The model under review builds one solid part; all positions refer to its coordinate system, in mm. A direction names the side the tool comes from. Coordinates: 2 decimals unless noted, no trailing zeros. Write each loop counter-clockwise with the first axis right and the second up, starting at its lowest first coordinate (ties: lowest second). Pieces come first, ordered by that corner, then holes. Notation, with made-up numbers: (84.5, 67.5) - (125.5, 67.5) arc R17 cw to (125.5, 86.5) - close; hole circle Ø7 at (-28.75, 41.5). An arc over 180 degrees is marked (long way). Put each result on its own line as item: value. Start each with the question number.
Item 1: Machinability: for faces 5 (the face through (-0.867, 3.905, -29.371)), 6 (the face through (-0.058, 0.466, -38.022)), 7 (the face through (0, 0, 10.5)), 8 (the face through (-0.867, -3.905, 6.444)), 9 (the face through (6.026, 10.438, 6.444)), which of the approach directions +Z, -Z, +X, -X, +Y, -Y give a long, thin tool a straight path to every point of the face, cutting with its end or side? Answer none if there is none.
Item 2: To check wall thickness, follow L1, parallel to Z at x = 0.5, y = 0; L2, parallel to Y at x = -0.25, z = -39.5; L3, parallel to Z at x = 4, y = 11.5. State the ranges of each line that lie inside material, in increasing order. Write a range as [from, to].
Item 3: Consider section A-A on y = 0. Give the boundary of the cut face in (x, z), then the cut area to 3 significant figures.
Item 4: Consider section D-D on z = -39.5. Give the boundary of the cut face in (x, y), then the cut area to 3 significant figures.
Item 5: Consider section C-C on z = -9.5. Give the boundary of the cut face in (x, y).
Item 6: Mouldability with a two-part tool opening along X and no side actions: class faces 1 (the face through (-5.974, 10.347, 6.444)), 2 (the face through (0.06, 8.25, 6.44)), 3 (the face through (-0.12, 15.75, 6.44)), 4 (the face through (0, 0, -55.5)) as pulls with the +X half, pulls with the -X half, needs draft (parallel to the pull), parting line crosses it, or undercut.
Item 7: Consider section B-B on x = 0. Give the boundary of the cut face in (y, z), then the cut area to 3 significant figures.
Item 8: For pin 1 (4 mm diameter, centred on x = 8, y = -0.5, fed in from +Z); pin 2 (6 mm diameter, centred on y = -4.5, z = 4, fed in from +X); pin 3 (8 mm diameter, centred on x = 6.5, z = -13, fed in from +Y), all flat-tipped, find the tip position at first contact; note any pin that passes through.
```python
from build123d import *

# Parameters (mm, degrees)
SKETCH1_R                           = 17.5
BOSS_EXTRUDE1_DEPTH                 = 2.5
BOSS_EXTRUDE2_DEPTH                 = 8
SKETCH3_R                           = 4
BOSS_EXTRUDE3_DEPTH                 = 8
BOSS_EXTRUDE4_START                 = 53
SKETCH7_R                           = 4
BOSS_EXTRUDE4_DEPTH                 = 53
CUT_EXTRUDE1_REACH                  = 62.768
CUT_EXTRUDE1_END_RADIUS             = 4
SKETCH8_R                           = 1.55
CUT_EXTRUDE1_DIRECTION_2_REACH      = 62.768
CUT_EXTRUDE1_DIRECTION_2_END_RADIUS = 4


with BuildPart() as part:
    # Sketch1 → Boss-Extrude1 (new, symmetric)
    with BuildSketch(Plane.XY):
        Circle(SKETCH1_R)
    extrude(amount=BOSS_EXTRUDE1_DEPTH, both=True)

    # Sketch2 → Boss-Extrude2 (add)
    with BuildSketch(Plane.XY.offset(2.5)):
        with BuildLine():
            Line((7.875, 13.63990011), (4.125, 7.144709581))
            ThreePointArc((4.125, 7.144709581), (0, 8.25), (-4.125, 7.144709581))
            Line((-4.125, 7.144709581), (-7.875, 13.63990011))
            ThreePointArc((-7.875, 13.63990011), (0, 15.75), (7.875, 13.63990011))
        make_face()
    extrude(amount=BOSS_EXTRUDE2_DEPTH)

    # Sketch3 → Boss-Extrude3 (add)
    with BuildSketch(Plane.XY.offset(2.5)):
        Circle(SKETCH3_R)
    extrude(amount=BOSS_EXTRUDE3_DEPTH)

    # Sketch7 → Boss-Extrude4 (add)
    with BuildSketch(Plane(origin=(0, 0, -2.5), x_dir=(-1, 0, 0), z_dir=(0, 0, -1)).offset(BOSS_EXTRUDE4_START)):
        with Locations(Location((0, 0, 0), (0, 0, 180))):
            Circle(SKETCH7_R)
    extrude(amount=-BOSS_EXTRUDE4_DEPTH)

    # Cut-Extrude1: up to this cylinder (the profile starts inside it)
    cut_extrude1_end = Plane(origin=(0, 0, -39.5), z_dir=(0, 0, 1)) * Cylinder(CUT_EXTRUDE1_END_RADIUS, 134.536, mode=Mode.PRIVATE)
    # Sketch8 → Cut-Extrude1 (cut, up to the surface)
    with BuildSketch(Plane.ZY, mode=Mode.PRIVATE) as cut_extrude1_sk1:
        with Locations((-39.5, 0)):
            Circle(SKETCH8_R)
    cut_extrude1_tool1 = extrude(cut_extrude1_sk1.sketch, amount=-CUT_EXTRUDE1_REACH, mode=Mode.PRIVATE) & cut_extrude1_end
    add(cut_extrude1_tool1.solids().sort_by_distance((0, 0, -39.5))[0], mode=Mode.SUBTRACT)

    # Cut-Extrude1 direction 2: up to this cylinder (the profile starts inside it)
    cut_extrude1_direction_2_end = Plane(origin=(0, 0, -39.5), z_dir=(0, 0, 1)) * Cylinder(CUT_EXTRUDE1_DIRECTION_2_END_RADIUS, 134.536, mode=Mode.PRIVATE)
    # Sketch8 → Cut-Extrude1 direction 2 (cut, up to the surface)
    with BuildSketch(Plane.ZY, mode=Mode.PRIVATE) as cut_extrude1_direction_2_sk1:
        with Locations((-39.5, 0)):
            Circle(SKETCH8_R)
    cut_extrude1_direction_2_tool1 = extrude(cut_extrude1_direction_2_sk1.sketch, amount=CUT_EXTRUDE1_DIRECTION_2_REACH, mode=Mode.PRIVATE) & cut_extrude1_direction_2_end
    add(cut_extrude1_direction_2_tool1.solids().sort_by_distance((0, 0, -39.5))[0], mode=Mode.SUBTRACT)


solid = part.part
```
Report:
1. face 5: -Z
1. face 6: +X, -X
1. face 7: +Z, +X, -X, +Y, -Y
1. face 8: +Z
1. face 9: +Z, +X, -Y
2. L1: [-55.5, -41.05], [-37.95, 10.5]
2. L2: [-3.99, -1.55], [1.55, 3.99]
2. L3: [-2.5, 10.5]
3. outline: (-17.5, -2.5) - (-4, -2.5) - (-4, -37.95) - (4, -37.95) - (4, -2.5) - (17.5, -2.5) - (17.5, 2.5) - (4, 2.5) - (4, 10.5) - (-4, 10.5) - (-4, 2.5) - (-17.5, 2.5) - close; (-4, -55.5) - (4, -55.5) - (4, -41.05) - (-4, -41.05) - close
3. area: 638 mm²
4. outline: (-3.69, -1.55) arc R4 ccw to (3.69, -1.55) - close; (-3.69, 1.55) - (3.69, 1.55) arc R4 ccw to start
4. area: 26.1 mm²
5. outline: circle Ø8 at (0, 0)
6. face 1: pulls with the -X half
6. face 2: undercut
6. face 3: parting line crosses it
6. face 4: needs draft
7. outline: (-17.5, -2.5) - (-4, -2.5) - (-4, -55.5) - (4, -55.5) - (4, -2.5) - (17.5, -2.5) - (17.5, 2.5) - (15.75, 2.5) - (15.75, 10.5) - (8.25, 10.5) - (8.25, 2.5) - (4, 2.5) - (4, 10.5) - (-4, 10.5) - (-4, 2.5) - (-17.5, 2.5) - close; hole circle Ø3.1 at (0, -39.5)
7. area: 715 mm²
8. pin 1: z = 2.5
8. pin 2: x = 17.4
8. pin 3: y = 3.12
